Part print with two shaded views. Sizes in mm from the minimum x, y, z corner. Coordinates: 2 decimals unless noted, no trailing zeros. Loops run counter-clockwise (first coordinate to the right, second up) from the corner with the lowest first, then second, coordinate; pieces in that order, holes last. Notation, with made-up numbers: (11, 0) -> (47, 0) arc R22 ccw to (47, 8) -> close; hole circle Ø6 at (23, -37). An arc over 180 degrees is marked (long way). Return JSON: item names as keys, results as strings. Group by question number.
(1) Saw through at C-C on x = 203. Write the cut outline in (y, z).
(2) Probe L1, parallel to X at y = 10.5, z = 9.5; L2, parallel to Y at x = 99, z = 9.75; L3, parallel to Z at x = 58, y = 16 (1 decimal). List the from-to ranges inside material, lowest first.
(3) Flat gauge pins, fed straight in: pin 1 Ø0.8 at (x, y) = (277.5, 22) entering from -Z; pin 2 Ø0.8 at (x, z) = (278, 22.5) entering from +Y; pin 3 Ø1.5 at (x, y) = (184.5, 14.5) entering from -Z; pin 4 Ø2 at (y, z) = (22.5, 22.5) entering from -X. Where does each tip first touch, or does it go through?
(4) Saw through at B-B on z = 4. Write the cut outline in (x, y).
(5) Saw through at A-A on y = 4.25. Write the cut outline in (x, z).
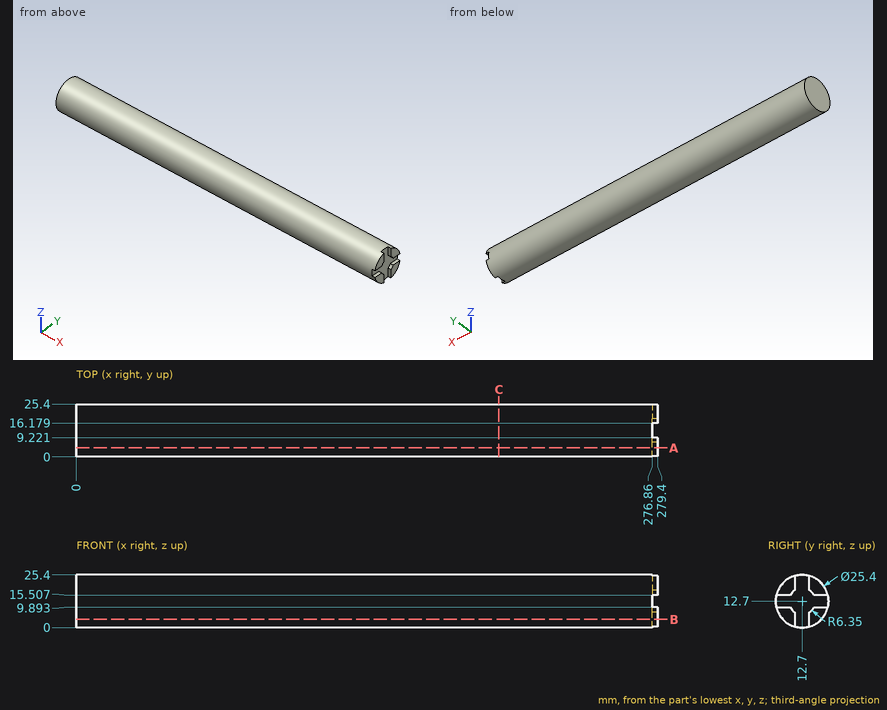
Geometry results:
{
 "1": {"outline": "circle Ø25.4 at (12.7, 12.7)"},
 "2": {"L1": "0 to 276.86", "L2": "0.35 to 25.05", "L3": "0.4 to 25"},
 "3": {"pin 1": "z = 3.64", "pin 2": "y = 21.24", "pin 3": "z = 0.04", "pin 4": "through"},
 "4": {"outline": "(0, 3.45) -> (279.4, 3.45) -> (279.4, 9.22) -> (276.86, 9.22) -> (276.86, 16.18) -> (279.4, 16.18) -> (279.4, 21.95) -> (0, 21.95) -> close"},
 "5": {"outline": "(0, 3.22) -> (279.4, 3.22) -> (279.4, 9.89) -> (276.86, 9.89) -> (276.86, 15.51) -> (279.4, 15.51) -> (279.4, 22.18) -> (0, 22.18) -> close"}
}
